Here's how the part is built. I have some questions about the finished solid (model axes, mm). Face numbers are marked on the shaded views. A direction names the side the tool comes from. Coordinates: 2 decimals unless noted, no trailing zeros. Write each loop counter-clockwise with the first axis right and the second up, starting at its lowest first coordinate (ties: lowest second). Pieces come first, ordered by that corner, then holes. Notation, with made-up numbers: (72, 10.5) - (93, 10.5) arc R13 cw to (93, 16.5) - close; hole circle Ø5 at (-25, -34). An arc over 180 degrees is marked (long way). Answer in a Markdown table with one row per item. Add a question column.
Item 1: We'd pull the mould along Y, two halves only. Please class the marked faces 1, 2 and 3: +Y half, -Y half, draft (parallel to the pull), parting line (faces both ways), or undercut.
Item 2: Imagine slicing it at B-B (x = 1.5). Please give me the cut outline in (y, z), plus the area to 3 significant figures.
Item 3: Which directions (+Z, -Z, +X, -X, +Y, -Y) give clear straight access to the entire face, cutting with the end or side of a thin tool? Please do the marked faces 4, 5, 6, 7 and 8.
Item 4: Imagine slicing it at C-C (z = 2.8). Please give me the cut outline in (x, y).
Item 5: Imagine slicing it at D-D (x = 9.25). Please give me the cut outline in (y, z).
Item 6: I'm going to push a flat-ended pin straight in: pin 1 (1.9 mm diameter, centred on x = 10, z = 2, fed in from +Y). Where does the tip first touch, or does it pass through?
Item 7: If I drill on probe 1 along X at (y, z) = (12.5, 0.8); probe 2 along Y at (x, z) = (4.5, 1.15); probe 3 along X at (y, z) = (8.25, 3.15), over which ranges is the centre line in solid material (lowest first)? Write a range as from..to.
Item 8: Imagine slicing it at A-A (y = 1.75). Please give me the cut outline in (x, z), plus the area to 3 significant figures.
Autodesk Fusion 360 part; units mm, degrees
sketch "Sketch1" plane through (0, 0, 0) normal (0, 0, 1) x (1, 0, 0)
  line L0 (0, 0) -> (20, 0)
  line L1 (20, 0) -> (20, 15)
  line L2 (20, 15) -> (0, 15)
  line L3 (0, 15) -> (0, 0)
  line L4 (15, 0) -> (15, 15)
  line L5 (5, 0) -> (5, 15)
  line L6 (0, 7.5) -> (20, 7.5) construction
  line L7 (0, 5.5) -> (20, 5.5)
  line L8 (0, 9.5) -> (20, 9.5)
  line L9 (10, 15) -> (10, 0) construction
  line L10 (8, 15) -> (8, 0)
  line L11 (12, 15) -> (12, 0)
  dimension "d1" = 2
  dimension "d2" = 2
extrude "Extrude1" add sketch "Sketch1" along normal blind 3.8 contours L0 L3 L5 L7 | L0 L5 L7 L10 | L5 L7 L8 L10 | L2 L3 L5 L8 | L0 L4 L7 L11 | L7 L8 L10 L11 | L2 L5 L8 L10 | L0 L1 L4 L7 | L4 L7 L8 L11 | L2 L4 L8 L11 | L1 L2 L4 L8
sketch "Sketch2" plane through (0, 0, 3.8) normal (0, 0, 1) x (-1, 0, 0)
  line L0 (-15, -5.5) -> (-15, -9.5)
  line L1 (-15, -9.5) -> (-20, -9.5)
  line L2 (-20, -9.5) -> (-20, -15)
  line L3 (-20, -15) -> (-12, -15)
  line L4 (-12, -15) -> (-12, -9.5)
  line L5 (-12, -9.5) -> (-8, -9.5)
  line L6 (-8, -9.5) -> (-8, -15)
  line L7 (-8, -15) -> (0, -15)
  line L8 (0, -15) -> (0, -9.5)
  line L9 (0, -9.5) -> (-5, -9.5)
  line L10 (-5, -9.5) -> (-5, -5.5)
  line L11 (-5, -5.5) -> (0, -5.5)
  line L12 (0, -5.5) -> (0, 0)
  line L13 (0, 0) -> (-8, 0)
  line L14 (-8, 0) -> (-8, -5.5)
  line L15 (-8, -5.5) -> (-12, -5.5)
  line L16 (-12, -5.5) -> (-12, 0)
  line L17 (-12, 0) -> (-20, 0)
  line L18 (-20, 0) -> (-20, -5.5)
  line L19 (-20, -5.5) -> (-15, -5.5)
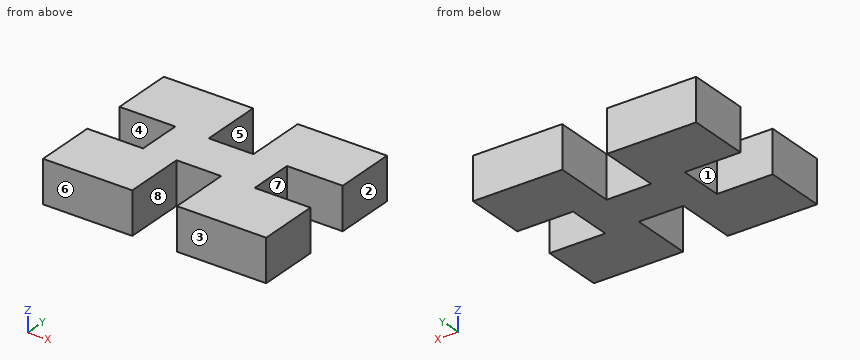
Here are the results:
| question | item | result |
|---|---|---|
| 1 | face 1 | undercut |
| 1 | face 2 | draft |
| 1 | face 3 | -Y half |
| 2 | outline | (0, 0) - (5.5, 0) - (5.5, 3.8) - (0, 3.8) - close; (9.5, 0) - (15, 0) - (15, 3.8) - (9.5, 3.8) - close |
| 2 | area | 41.8 mm2 |
| 3 | face 4 | +Z, -Z, -X |
| 3 | face 5 | +Z, -Z, +Y |
| 3 | face 6 | +Z, -Z, +X, -X, -Y |
| 3 | face 7 | +Z, -Z, +X |
| 3 | face 8 | +Z, -Z, -Y |
| 4 | outline | (0, 0) - (8, 0) - (8, 5.5) - (12, 5.5) - (12, 0) - (20, 0) - (20, 5.5) - (15, 5.5) - (15, 9.5) - (20, 9.5) - (20, 15) - (12, 15) - (12, 9.5) - (8, 9.5) - (8, 15) - (0, 15) - (0, 9.5) - (5, 9.5) - (5, 5.5) - (0, 5.5) - close |
| 5 | outline | (5.5, 0) - (9.5, 0) - (9.5, 3.8) - (5.5, 3.8) - close |
| 6 | pin 1 | stops at y = 9.5 |
| 7 | probe 1 | x = 0..8, 12..20 |
| 7 | probe 2 | y = 0..5.5, 9.5..15 |
| 7 | probe 3 | x = 5..15 |
| 8 | outline | (0, 0) - (8, 0) - (8, 3.8) - (0, 3.8) - close; (12, 0) - (20, 0) - (20, 3.8) - (12, 3.8) - close |
| 8 | area | 60.8 mm2 |
